```python
from build123d import *

# Parameters (mm, degrees)
SKETCH1_W              = 106
SKETCH1_H              = 106
SKETCH1_W_2            = 102
SKETCH1_H_2            = 102
BOSS_EXTRUDE1_DEPTH    = 140
SKETCH2_W              = 155
SKETCH2_H              = 145
BOSS_EXTRUDE2_DEPTH    = 2
SKETCH3_R              = 5
CUT_EXTRUDE1_DEPTH     = 2
CUT_EXTRUDE2_START     = -131.5
CUT_EXTRUDE2_DEPTH     = 157
LPATTERN1_COUNT        = 2
LPATTERN1_PITCH        = 50
LPATTERN1_START        = -131.5
LPATTERN1_COPY_1_DEPTH = 157
FILLET1_R              = 2


with BuildPart() as part:
    # Sketch1 → Boss-Extrude1 (new body)
    with BuildSketch(Plane(origin=(0, 0, 0), x_dir=(1, 0, 0), z_dir=(0, 1, 0))):
        Rectangle(SKETCH1_W, SKETCH1_H)
        Rectangle(SKETCH1_W_2, SKETCH1_H_2, mode=Mode.SUBTRACT)
    extrude(amount=BOSS_EXTRUDE1_DEPTH)

    # Sketch2 → Boss-Extrude2 (add)
    with BuildSketch(Plane(origin=(0, 0, 0), x_dir=(1, 0, 0), z_dir=(0, 1, 0))):
        Rectangle(SKETCH2_W, SKETCH2_H)
    extrude(amount=BOSS_EXTRUDE2_DEPTH)

    # Sketch3 → Cut-Extrude1 (cut)
    with BuildSketch(Plane(origin=(0, 2, 0), x_dir=(1, 0, 0), z_dir=(0, 1, 0))):
        with Locations((-65, 61.040230774)):
            Circle(SKETCH3_R)
        with Locations((65, 61.040230774)):
            Circle(SKETCH3_R)
        with Locations((65, -60)):
            Circle(SKETCH3_R)
        with Locations((-65, -60)):
            Circle(SKETCH3_R)
    extrude(amount=-CUT_EXTRUDE1_DEPTH, mode=Mode.SUBTRACT)

    # Sketch4 → Cut-Extrude2 (cut)
    with BuildSketch(Plane(origin=(53, 0, 0), x_dir=(0, 0, -1), z_dir=(1, 0, 0)).offset(CUT_EXTRUDE2_START)):
        with BuildLine():
            Line((-23, 80), (-27, 80))
            ThreePointArc((-27, 80), (-28.414213562, 80.585786438), (-29, 82))
            Line((-29, 82), (-29, 118))
            ThreePointArc((-29, 118), (-28.414213562, 119.414213562), (-27, 120))
            Line((-27, 120), (-23, 120))
            ThreePointArc((-23, 120), (-21.585786438, 119.414213562), (-21, 118))
            Line((-21, 118), (-21, 82))
            ThreePointArc((-21, 82), (-21.585786438, 80.585786438), (-23, 80))
        make_face()
    cut_extrude2 = extrude(amount=CUT_EXTRUDE2_DEPTH, mode=Mode.SUBTRACT)

    # Mirror1: Cut-Extrude2 across plane
    add(cut_extrude2.mirror(Plane.XY), mode=Mode.SUBTRACT)

    # LPattern1: Cut-Extrude2 ×2
    with Locations(*[(0, -i * LPATTERN1_PITCH, 0) for i in range(1, LPATTERN1_COUNT)]):
        add(cut_extrude2, mode=Mode.SUBTRACT)

    # LPattern1 copy 1 sketch → LPattern1 copy 1 (cut)
    with BuildSketch(Plane(origin=(53, -50, 0), x_dir=(0, 0, 1), z_dir=(1, 0, 0)).offset(LPATTERN1_START)):
        with BuildLine():
            Line((-23, -80), (-27, -80))
            ThreePointArc((-27, -80), (-28.414213562, -80.585786438), (-29, -82))
            Line((-29, -82), (-29, -118))
            ThreePointArc((-29, -118), (-28.414213562, -119.414213562), (-27, -120))
            Line((-27, -120), (-23, -120))
            ThreePointArc((-23, -120), (-21.585786438, -119.414213562), (-21, -118))
            Line((-21, -118), (-21, -82))
            ThreePointArc((-21, -82), (-21.585786438, -80.585786438), (-23, -80))
        make_face()
    extrude(amount=LPATTERN1_COPY_1_DEPTH, mode=Mode.SUBTRACT)

    # Fillet1
    fillet1_edges = [part.edges().sort_by_distance(p)[0] for p in [
        (-51, 71, -51),
        (-51, 71, 51),
        (51, 71, 51),
        (51, 71, -51),
        (-53, 71, -53),
        (53, 71, -53),
        (53, 71, 53),
        (-53, 71, 53),
    ]]
    fillet(fillet1_edges, radius=FILLET1_R)


solid = part.part
```
Read the model definition and answer for the solid it produces. Units are mm, in the model's axes. A direction names the side the tool comes from. Round coordinates to 2 decimals unless told otherwise and drop trailing zeros. Write each loop counter-clockwise with the first axis right and the second up, starting at its lowest first coordinate (ties: lowest second). Pieces come first, ordered by that corner, then holes. Notation, with made-up numbers: (25, -4.75) - (32, -4.75) arc R6 cw to (32, 6.25) - close; hole circle Ø4 at (40, -31). An arc over 180 degrees is marked (long way). One line per item, written item: value.
Q1. Each of these flat-tipped pins is pushed along its axis until it touches: P1, Ø10, axis at y = 89, z = 55, coming from the -X side; P2, Ø1, axis at x = 35.5, z = -31, coming from the +Y side; P3, Ø0.6, axis at x = -51.5, y = 41.5, coming from the +Z side. Where does it stop, or does it pass through?
The answers:
P1: stops at x = -53
P2: stops at y = 2
P3: stops at z = 52.99
Q2. Find section A-A (x = 65). Determine the outline of the cut face in (y, z), and give its area (3 significant figures).
The answers:
outline: (0, -72.5) - (2, -72.5) - (2, -66.04) - (0, -66.04) - close; (0, -56.04) - (2, -56.04) - (2, 55) - (0, 55) - close; (0, 65) - (2, 65) - (2, 72.5) - (0, 72.5) - close
area: 250 mm2
Q3. Find section C-C (y = 43.5). Count the separate pieces of the cut face and the enclosed holes in it, and give its area (3 significant figures).
The answers:
separate pieces: 4
enclosed holes: 0
area: 768 mm2
Q4. Which of the six approach directions +Z, -Z, +X, -X, +Y, -Y give full straight-line access (tool end or side, diameter ignored) to faces 1 (the flat face through (-1, 70, -53)), 2 (the cylindrical face through (-65.651, 1.014, 55.043)), 3 (the flat face through (-51, 70, 1)), 4 (the flat face through (-53, 70, 1))?
The answers:
face 1: -Z, +X, -X, +Y
face 2: +Y, -Y
face 3: +Y
face 4: +Z, -Z, -X, +Y
Q5. Find section D-D (z = -42). Determine the outline of the cut face in (x, y).
The answers:
outline: (-77.5, 0) - (77.5, 0) - (77.5, 2) - (53, 2) - (53, 140) - (51, 140) - (51, 2) - (-51, 2) - (-51, 140) - (-53, 140) - (-53, 2) - (-77.5, 2) - close
Q6. Find section B-B (z = 60). Determine the outline of the cut face in (x, y), and give its area (3 significant figures).
The answers:
outline: (-77.5, 0) - (-70, 0) - (-70, 2) - (-77.5, 2) - close; (-60, 0) - (60, 0) - (60, 2) - (-60, 2) - close; (70, 0) - (77.5, 0) - (77.5, 2) - (70, 2) - close
area: 270 mm2
Q7. For a pull along Z with two mould halves and no side action, classify faces 5 (the flat face through (-1, 70, 53)), 6 (the cylindrical face through (-66.08, 1.01, -56.16)), 7 (the cylindrical face through (63.92, 1.01, -56.16)), 8 (the flat face through (53, 70, 1)) as pulls with the +Z half, pulls with the -Z half, needs draft (parallel to the pull), parting line crosses it, or undercut.
The answers:
face 5: pulls with the +Z half
face 6: undercut
face 7: undercut
face 8: needs draft
Q8. Straight lines are drawn through the part: line 1 (Z direction, x = 65, y = 1.4); line 2 (X direction, y = 96.5, z = 34.5); line 3 (X direction, y = 1, z = 60). For each, find the intervals that lie inside material, in ascending order. Write a range as from..to.
The answers:
line 1: z = -72.5..-66.04, -56.04..55, 65..72.5
line 2: x = -53..-51, 51..53
line 3: x = -77.5..-70, -60..60, 70..77.5
